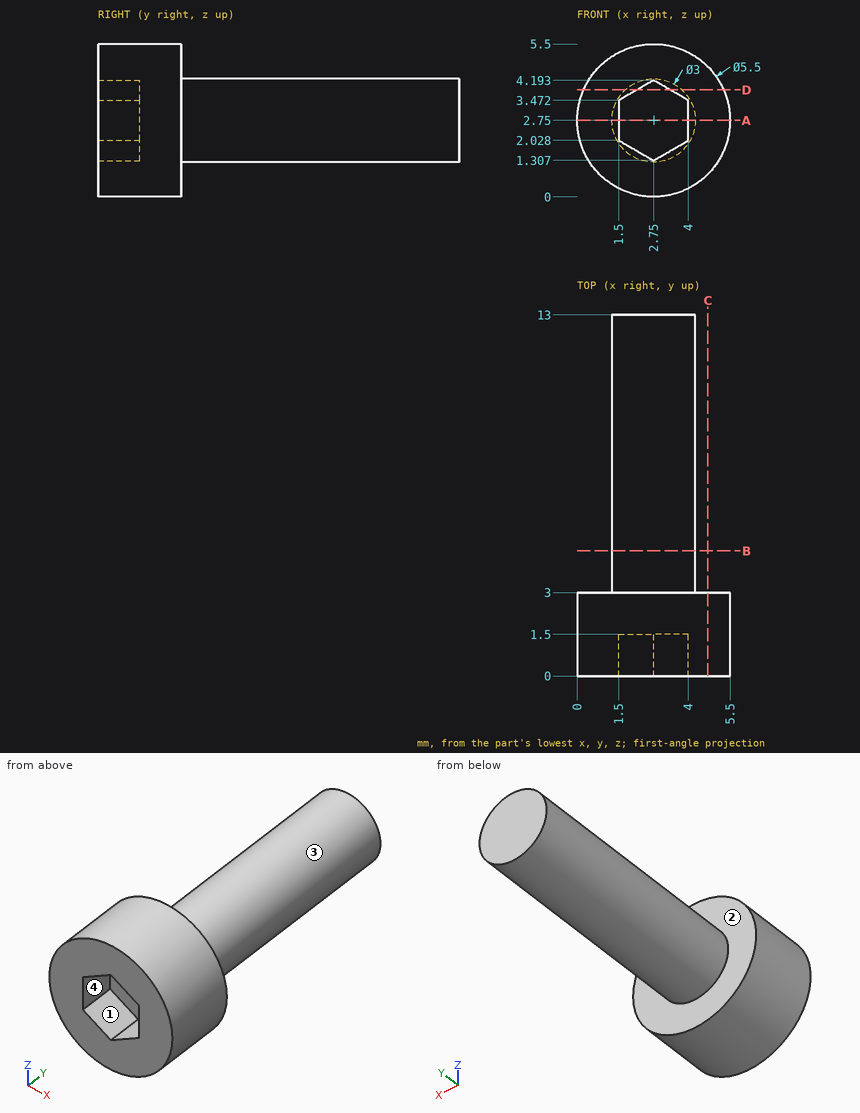
Geometry: see drawing. Coordinates: mm, zero at the bounding-box minimum. Coordinates: 2 decimals unless noted, no trailing zeros. Loops run counter-clockwise (first coordinate to the right, second up) from the corner with the lowest first, then second, coordinate; pieces in that order, holes last.
Q1. Cut plane D-D (z = 3.85). Output: boundary loops of the cut face in (x, y) (1 decimal).
Q2. Cut plane B-B (y = 4.5). Output: boundary loops of the cut face in (x, z).
Q3. Contact query for a flat-ended pin moving along its axis: pin 1 (1.5 mm diameter, centred on y = 6.5, z = 4.5, fed in from +X). Output: stop coordinate, or through.
Q4. Draft query along Z for the marked faces 1, 2, 3 and 4. Return one class per face: +Z half, -Z half, draft (parallel to the pull), parting line (faces both ways), or undercut.
Q5. Material intervals for line 1 (Y direction, x = 2.7, z = 1.8); line 2 (Y direction, x = 2.1, z = 4.4); line 3 (Z direction, x = 3.95, y = 1) (1 decimal), sorted ascending.
Q6. Cut plane C-C (x = 4.7). Output: boundary loops of the cut face in (y, z), then the cut area to 3 significant figures.
Q7. Cut plane A-A (z = 2.75). Output: boundary loops of the cut face in (x, y).
Working result:
1. outline: (0.2, 0) - (2.2, 0) - (2.2, 1.5) - (3.3, 1.5) - (3.3, 0) - (5.3, 0) - (5.3, 3) - (3.8, 3) - (3.8, 13) - (1.7, 13) - (1.7, 3) - (0.2, 3) - close
2. outline: circle Ø3 at (2.75, 2.75)
3. pin 1: stops at x = 3.87
4. face 1: undercut
4. face 2: draft
4. face 3: parting line
4. face 4: undercut
5. line 1: y = 1.5 to 13
5. line 2: y = 0 to 3
5. line 3: z = 0.3 to 2, 3.5 to 5.2
6. outline: (0, 0.81) - (3, 0.81) - (3, 4.69) - (0, 4.69) - close
6. area: 11.6 mm2
7. outline: (0, 0) - (1.5, 0) - (1.5, 1.5) - (4, 1.5) - (4, 0) - (5.5, 0) - (5.5, 3) - (4.25, 3) - (4.25, 13) - (1.25, 13) - (1.25, 3) - (0, 3) - close
